Here's the drawing with two shaded views (mm, measured from the low corner). I have some questions. A direction names the side the tool comes from. Coordinates: 2 decimals unless noted, no trailing zeros. Write each loop counter-clockwise with the first axis right and the second up, starting at its lowest first coordinate (ties: lowest second). Pieces come first, ordered by that corner, then holes.
Item 1: If we section it at B-B (y = 8): Please give me the cut outline in (x, z).
Item 2: For the marked faces 1 and 2, which set-ups out of +Z, -Z, +X, -X, +Y, -Y let a thin tool reach every point of the face, with its end or its side?
Item 3: If we section it at C-C (x = 2.75): Please give me the cut outline in (y, z), then the cut area to 3 significant figures.
Item 4: I'm going to push a flat-ended pin straight in: pin 1 Ø5 at (y, z) = (13.5, 6.5) entering from -X. Where does the tip first touch, or does it pass through?
Item 5: If we section it at D-D (y = 3): Please give me the cut outline in (x, z), then the cut area to 3 significant figures.
Item 6: If we section it at A-A (z = 10): Please give me the cut outline in (x, y).
Item 7: If I drill on line 1 (X direction, y = 7.75, z = 4.25); line 2 (Z direction, x = 3.25, y = 9); line 3 (Z direction, x = 5, y = 8.5), over which ranges is the centre line in solid material (lowest first)?
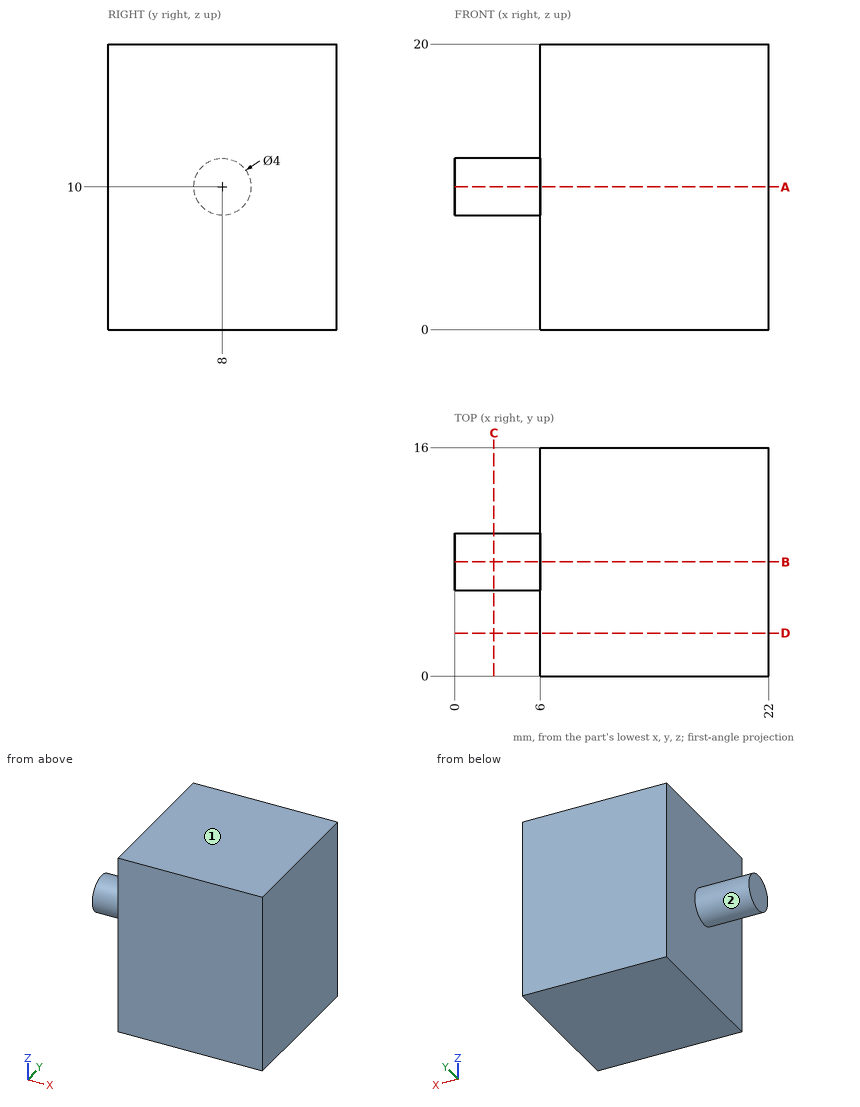
Answer list:
1. outline: (0, 8) - (6, 8) - (6, 0) - (22, 0) - (22, 20) - (6, 20) - (6, 12) - (0, 12) - close
2. face 1: +Z, +X, -X, +Y, -Y
2. face 2: -X
3. outline: circle Ø4 at (8, 10)
3. area: 12.6 mm2
4. pin 1: stops at x = 6
5. outline: (6, 0) - (22, 0) - (22, 20) - (6, 20) - close
5. area: 320 mm2
6. outline: (0, 6) - (6, 6) - (6, 0) - (22, 0) - (22, 16) - (6, 16) - (6, 10) - (0, 10) - close
7. line 1: x = 6 to 22
7. line 2: z = 8.27 to 11.73
7. line 3: z = 8.06 to 11.94
